Work out the finished part from the listing and answer in its coordinate system (mm). Face numbers are marked on the shaded views. A direction names the side the tool comes from. Coordinates: 2 decimals unless noted, no trailing zeros. Order: outer loops, then holes, each group sorted by start corner. A loop starts at its lowest first (then second) coordinate and runs counter-clockwise, first axis right, second up. Notation, with made-up numbers: (51.5, 4) - (109.5, 4) arc R21 ccw to (109.5, 43) - close; hole circle Ø6 at (79, 81.5). An arc over 180 degrees is marked (long way). Answer as a JSON object with one key per item and string values. Group by question number.
1) Each of these flat-tipped pins is pushed along its axis until it touches: P1, Ø2, axis at y = 15.5, z = 15, coming from the +X side; P2, Ø2, axis at y = 46.5, z = 16, coming from the -X side; P3, Ø18, axis at x = -2, y = 27, coming from the +Z side. Where does it stop, or does it pass through?
2) Section A-A (y = 31) is taken. Give the vertices of the cut face in (x, z), plus the area to 3 significant figures.
3) Section B-B (x = 0) is taken. Count the separate pieces of the cut face and the enclosed holes in it, plus the area to 3 significant figures.
4) The mould has two halves that part along X. Classify the marked faces 4, 5 and 6: released by +X, released by -X, zero draft, split by the parting line, or undercut.
5) Find the intervals of material crossed by line 1 along Y through (x, z) = (0, 29); line 2 along Z through (x, y) = (-10, 38.5); line 3 along Y through (x, z) = (0, 37.25), in increasing order.
6) A tool of negligible diameter and unlimited length cuts with its end or side. For the marked faces 1, 2 and 3, from which of +Z, -Z, +X, -X, +Y, -Y can it reach the whole face along a straight path? Write none if from no direction.
7) Section C-C (y = 41) is taken. Give the vertices of the cut face in (x, z), plus the area to 3 significant figures.
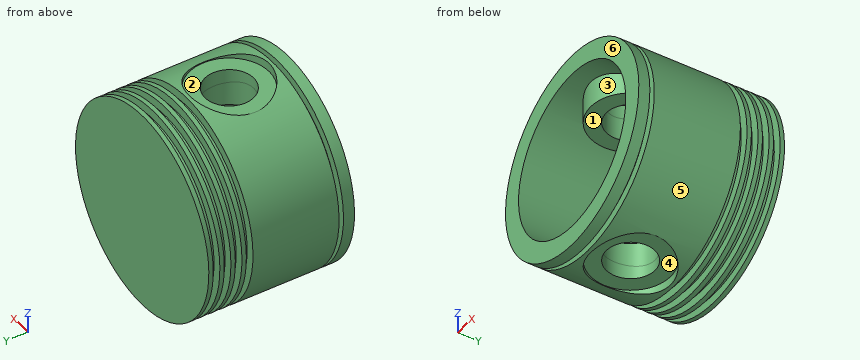
from build123d import *

# Parameters (mm, degrees)
CUT_EXTRUDE1_DEPTH       = 93.671462706
CUT_EXTRUDE1_DEPTH_BACK  = 93.671462706
SKETCH2_R                = 11
BOSS_EXTRUDE1_REACH      = 119.671
BOSS_EXTRUDE1_END_RADIUS = 37
BOSS_EXTRUDE1_START      = 25
SKETCH2_3_R              = 18
SKETCH2_3_R_2            = 11
CUT_EXTRUDE3_START       = 42
SKETCH2_5_R              = 18
SKETCH2_5_R_2            = 11
CUT_EXTRUDE3_DEPTH       = 4


with BuildPart() as part:
    # Sketch1 → Revolve1 (revolve)
    with BuildSketch(Plane.XY, mode=Mode.PRIVATE) as revolve1_sk:
        Polygon((0, 66), (46, 66), (46, 64), (42, 64), (42, 61), (46, 61), (46, 59), (42, 59), (42, 56), (46, 56), (46, 54), (42, 54), (42, 51), (46, 51), (46, 49), (42, 49), (42, 46), (46, 46), (46, 7), (42, 7), (42, 5), (46, 5), (46, 0), (37, 0), (37, 62), (0, 62), align=None)
    revolve(revolve1_sk.sketch.rotate(Axis((0, 0, 0), (0, 1, 0)), 90), axis=Axis((0, 0, 0), (0, 1, 0)))

    # Sketch2 → Cut-Extrude1 (cut, two sides: drawn at the far end of the back side and taken through both)
    with BuildSketch(Plane.XY.offset(-CUT_EXTRUDE1_DEPTH_BACK)):
        with Locations((0, 26.5)):
            Circle(SKETCH2_R)
    extrude(amount=CUT_EXTRUDE1_DEPTH + CUT_EXTRUDE1_DEPTH_BACK, mode=Mode.SUBTRACT)

    # Boss-Extrude1: up to this cylinder (the profile starts inside it)
    boss_extrude1_end = Plane(origin=(0, 26.5, 0), z_dir=(0, -1, 0)) * Cylinder(BOSS_EXTRUDE1_END_RADIUS, 314.342, mode=Mode.PRIVATE)
    # Sketch2<3> → Boss-Extrude1 (add, up to the surface)
    with BuildSketch(Plane.XY.offset(BOSS_EXTRUDE1_START), mode=Mode.PRIVATE) as boss_extrude1_sk1:
        with Locations(Location((0, 26.5, 0), (0, 0, 180))):
            Circle(SKETCH2_3_R)
        with Locations((0, 26.5)):
            Circle(SKETCH2_3_R_2, mode=Mode.SUBTRACT)
    boss_extrude1_tool1 = extrude(boss_extrude1_sk1.sketch, amount=BOSS_EXTRUDE1_REACH, mode=Mode.PRIVATE) & boss_extrude1_end
    boss_extrude1 = boss_extrude1_tool1.solids().sort_by_distance((17.490883, 26.5, 25))[0]
    add(boss_extrude1)

    # Sketch2<5> → Cut-Extrude3 (cut)
    with BuildSketch(Plane.XY.offset(CUT_EXTRUDE3_START)):
        with Locations(Location((0, 26.5, 0), (0, 0, 180))):
            Circle(SKETCH2_5_R)
        with Locations((0, 26.5)):
            Circle(SKETCH2_5_R_2, mode=Mode.SUBTRACT)
    cut_extrude3 = extrude(amount=CUT_EXTRUDE3_DEPTH, mode=Mode.SUBTRACT)

    # Mirror1: Boss-Extrude1, Cut-Extrude3 across plane
    add(boss_extrude1.mirror(Plane.XY))
    add(cut_extrude3.mirror(Plane.XY), mode=Mode.SUBTRACT)


solid = part.part
Report:
{
 "1": {"P1": "stops at x = 43.82", "P2": "stops at x = -43.44", "P3": "stops at z = 42"},
 "2": {"outline": "(-17.43, -42.57) - (-17.43, -42) - (-10.04, -42) - (-10.04, -25) - (-17.43, -25) - (-17.43, -32.64) arc R37 cw to (-17.43, 32.64) - (-17.43, 25) - (-10.04, 25) - (-10.04, 42) - (-17.43, 42) - (-17.43, 42.57) arc R46 ccw to start; (10.04, -42) - (17.43, -42) - (17.43, -42.57) arc R46 ccw to (17.43, 42.57) - (17.43, 42) - (10.04, 42) - (10.04, 25) - (17.43, 25) - (17.43, 32.64) arc R37 cw to (17.43, -32.64) - (17.43, -25) - (10.04, -25) - close", "area": "2,200 mm²"},
 "3": {"separate pieces": "3", "enclosed holes": "0", "area": "1,200 mm²"},
 "4": {"face 4": "undercut", "face 5": "split by the parting line", "face 6": "zero draft"},
 "5": {"line 1": "y = 8.5 to 15.5, 37.5 to 44.5, 62 to 66", "line 2": "z = -42 to -25, 25 to 42", "line 3": "y = 0 to 15.5, 37.5 to 66"},
 "6": {"face 1": "-Y", "face 2": "+Z", "face 3": "none"},
 "7": {"outline": "(-10.67, -44.75) - (-10.67, -42) - (10.67, -42) - (10.67, -44.75) arc R46 ccw to (10.67, 44.75) - (10.67, 42) - (-10.67, 42) - (-10.67, 44.75) arc R46 ccw to start; hole (-10.67, -35.43) - (-10.67, -25) - (10.67, -25) - (10.67, -35.43) arc R37 ccw to (10.67, 35.43) - (10.67, 25) - (-10.67, 25) - (-10.67, 35.43) arc R37 ccw to start", "area": "2,680 mm²"}
}
